Autodesk Inventor part; units mm, degrees
ref_plane "YZ Plane" through (0, 0, 0) normal (1, 0, 0) x (0, 1, 0)
ref_plane "XZ Plane" through (0, 0, 0) normal (0, 1, 0) x (-1, 0, 0)
ref_plane "XY Plane" through (0, 0, 0) normal (0, 0, 1) x (1, 0, 0)
sketch "Sketch1" plane through (0, 0, 0) normal (0, 0, 1) x (1, 0, 0)
  circle A0 centre (0, 0) radius 15.875
  line L0 (7.8823, 1.8652) -> (9.8245, 1.8652)
  arc A1 (9.7695, -2.1348) -> (9.8245, 1.8652) centre (0, 0) ccw
  line L1 (9.7695, -2.1348) -> (7.8136, -2.1348)
  arc A2 (5.5564, -5.8937) -> (7.8136, -2.1348) centre (0, 0) ccw
  line L2 (5.5564, -5.8937) -> (6.5275, -7.5757)
  arc A3 (3.0359, -9.528) -> (6.5275, -7.5757) centre (0, 0) ccw
  line L3 (3.0359, -9.528) -> (2.058, -7.8342)
  arc A4 (-2.3259, -7.7589) -> (2.058, -7.8342) centre (0, 0) ccw
  line L4 (-2.3259, -7.7589) -> (-3.297, -9.4409)
  arc A5 (-6.7336, -7.3932) -> (-3.297, -9.4409) centre (0, 0) ccw
  line L5 (-6.7336, -7.3932) -> (-5.7556, -5.6994)
  arc A6 (-7.8823, -1.8652) -> (-5.7556, -5.6994) centre (0, 0) ccw
  line L6 (-7.8823, -1.8652) -> (-9.8245, -1.8652)
  arc A7 (-9.7695, 2.1348) -> (-9.8245, -1.8652) centre (0, 0) ccw
  line L7 (-9.7695, 2.1348) -> (-7.8136, 2.1348)
  arc A8 (-5.5564, 5.8937) -> (-7.8136, 2.1348) centre (0, 0) ccw
  line L8 (-5.5564, 5.8937) -> (-6.5275, 7.5757)
  arc A9 (-3.0359, 9.528) -> (-6.5275, 7.5757) centre (0, 0) ccw
  line L9 (-3.0359, 9.528) -> (-2.058, 7.8342)
  arc A10 (2.3259, 7.7589) -> (-2.058, 7.8342) centre (0, 0) ccw
  line L10 (2.3259, 7.7589) -> (3.297, 9.4409)
  arc A11 (6.7336, 7.3932) -> (3.297, 9.4409) centre (0, 0) ccw
  line L11 (6.7336, 7.3932) -> (5.7556, 5.6994)
  arc A12 (7.8823, 1.8652) -> (5.7556, 5.6994) centre (0, 0) ccw
extrude "Extrusion1" add sketch "Sketch1" along normal blind 6.35
properties part number "coupler window motor"
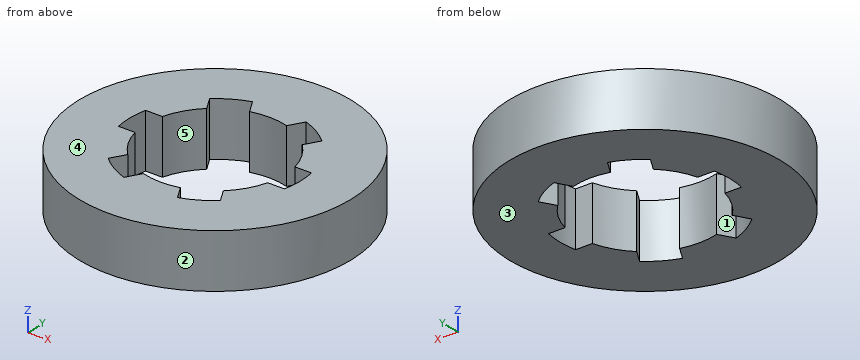
Source: CAD feature listing. Evaluate the final solid. Frame: model axes, mm. Face numbers are marked on the shaded views. A direction names the side the tool comes from. Round coordinates to 2 decimals unless told otherwise and drop trailing zeros. Loops run counter-clockwise (first coordinate to the right, second up) from the corner with the lowest first, then second, coordinate; pieces in that order, holes last. Notation, with made-up numbers: (33, 47.5) - (60, 47.5) arc R27 ccw to (60, 66.5) - close; hole circle Ø7 at (-31.5, 76.25). An arc over 180 degrees is marked (long way). Write item = value, one per line. Start each with the question number.
Item 1: Section query A-A on y = 0. Output: boundary loops of the cut face in (x, z) (3 decimals), plus the area to 3 significant figures.
Item 2: Material intervals for line 1 (X direction, y = 9, z = 2.25); line 2 (Y direction, x = 2, z = 2.5); line 3 (Y direction, x = 4, z = 3.75), sorted ascending.
Item 3: Section query D-D on y = 13. Output: boundary loops of the cut face in (x, z), plus the area to 3 significant figures.
Item 4: Section query B-B on x = 0. Output: boundary loops of the cut face in (y, z) (3 decimals), plus the area to 3 significant figures.
Item 5: Reachability of the marked faces 4 and 5 from +Z, -Z, +X, -X, +Y, -Y: full face, straight path, thin tool, end or side. Return the list, or none.
Item 6: First-contact query: pin 1 Ø1.5 at (x, z) = (-5, 2.5) entering from -Y; pin 2 Ø1.6 at (x, z) = (9, 2) entering from +Y; pin 3 Ø1 at (x, z) = (-8.5, 3.5) entering from -Y. Flat tips, straight axial feed; report the tip coordinate or a pass-through.
Item 7: Mould query, pull axis X, two halves, no side actions, for the marked faces 1, 2 and 3. Classes: released by +X, released by -X, zero draft, split by the parting line, or undercut.
Results list:
q1.outline = (-15.875, 0) - (-10, 0) - (-10, 6.35) - (-15.875, 6.35) - close; (10, 0) - (15.875, 0) - (15.875, 6.35) - (10, 6.35) - close
q1.area = 74.6 mm²
q2.line_1 = -13.08 to -4.36, -2.73 to 3.04, 4.36 to 13.08
q2.line_2 = -15.75 to -7.85, 7.85 to 15.75
q2.line_3 = -15.36 to -9.17, 9.17 to 15.36
q3.outline = (-9.11, 0) - (9.11, 0) - (9.11, 6.35) - (-9.11, 6.35) - close
q3.area = 116 mm²
q4.outline = (-15.875, 0) - (-8.1, 0) - (-8.1, 6.35) - (-15.875, 6.35) - close; (8.1, 0) - (15.875, 0) - (15.875, 6.35) - (8.1, 6.35) - close
q4.area = 98.7 mm²
q5.face_4 = +Z, +X, -X, +Y, -Y
q5.face_5 = +Z, -Z
q6.pin_1 = -15.3
q6.pin_2 = 13.59
q6.pin_3 = -13.71
q7.face_1 = undercut
q7.face_2 = split by the parting line
q7.face_3 = zero draft
